```python
from build123d import *

# Parameters (mm, degrees)
SKETCH1_R                    = 14
BOSS_EXTRUDE1_DEPTH          = 10
SKETCH2_R                    = 6
CUT_EXTRUDE1_DEPTH           = 23.181073013
SKETCH3_R                    = 1.5
CUT_EXTRUDE2_DEPTH           = 23.181073013
CHAMFER1_SIZE                = 0.8
CHAMFER2_SIZE                = 0.3
CIRPATTERN1_COUNT            = 3
CHAMFER2_OF_CIRPATTERN1_SIZE = 0.3


with BuildPart() as part:
    # Sketch1 → Boss-Extrude1 (new body)
    with BuildSketch(Plane(origin=(0, 0, 0), x_dir=(1, 0, 0), z_dir=(0, 1, 0))):
        with Locations(Location((0, 0, 0), (0, 0, 270))):
            Circle(SKETCH1_R)
    extrude(amount=BOSS_EXTRUDE1_DEPTH)

    # Sketch2 → Cut-Extrude1 (cut, through all)
    with BuildSketch(Plane(origin=(0, 10, 0), x_dir=(1, 0, 0), z_dir=(0, 1, 0))):
        with Locations(Location((0, 0, 0), (0, 0, 270))):
            Circle(SKETCH2_R)
    extrude(amount=-CUT_EXTRUDE1_DEPTH, mode=Mode.SUBTRACT)

    # Sketch3 → Cut-Extrude2 (cut, through all)
    with BuildSketch(Plane(origin=(0, 10, 0), x_dir=(1, 0, 0), z_dir=(0, 1, 0))):
        with Locations(Location((0, 10.5, 0), (0, 0, 270))):
            Circle(SKETCH3_R)
    cut_extrude2 = extrude(amount=-CUT_EXTRUDE2_DEPTH, mode=Mode.SUBTRACT)

    # Chamfer1
    chamfer1_edges = [part.edges().sort_by_distance(p)[0] for p in [
        (0, 0, -14),
        (0, 10, -14),
        (0, 0, -6),
        (0, 10, -6),
    ]]
    chamfer(chamfer1_edges, length=CHAMFER1_SIZE)

    # Chamfer2
    chamfer2_edges = [part.edges().sort_by_distance(p)[0] for p in [
        (0, 0, -12),
        (0, 10, -12),
    ]]
    chamfer(chamfer2_edges, length=CHAMFER2_SIZE)

    # CirPattern1: Cut-Extrude2 ×3 about axis
    cirpattern1_axis = Axis((0, 0, 0), (0, 1, 0))
    for i in range(1, CIRPATTERN1_COUNT):
        add(cut_extrude2.rotate(cirpattern1_axis, i * 360 / CIRPATTERN1_COUNT), mode=Mode.SUBTRACT)

    # Chamfer2 of CirPattern1
    chamfer2_of_cirpattern1_edges = [part.edges().sort_by_distance(p)[0] for p in [
        (-10.392304845, 0, 6),
        (-10.392304845, 10, 6),
        (10.392304845, 0, 6),
        (10.392304845, 10, 6),
    ]]
    chamfer(chamfer2_of_cirpattern1_edges, length=CHAMFER2_OF_CIRPATTERN1_SIZE)


solid = part.part
```
Source: CAD feature listing. Evaluate the final solid. Frame: model axes, mm. Give positions to 0.01 mm unless a question says otherwise; leave off trailing zeros. Order: outer loops, then holes, each group sorted by start corner. A loop starts at its lowest first (then second) coordinate and runs counter-clockwise, first axis right, second up.
(1) Material intervals for line 1 along Z through (x, y) = (0.5, 8); line 2 along X through (y, z) = (6.25, 5.5); line 3 along Z through (x, y) = (-3.75, 6.5), sorted ascending.
(2) Section query C-C (y = 3.5). Return the cut outline in (x, z).
(3) Contact query for flat-ended pins moving along their axis: P1, Ø4, axis at y = 8.5, z = -8.5, coming from the -X side; P2, Ø2, axis at x = 6, y = 4.5, coming from the +Z side; P3, Ø3, axis at y = 2.5, z = 2, coming from the -X side; P4, Ø2.5, axis at x = 0, z = -10.5, coming from the +Y side. Output: stop coordinate, or through.
(4) Section query B-B (x = 0). Return the cut outline in (y, z), plus the area to 3 significant figures.
(5) Section query A-A (z = 0). Return the cut outline in (x, y).
(6) Section query D-D (z = 5.25). State how many separate pieces and enclosed holes the cut face has, plus the area to 3 significant figures.
(7) Pull-direction query (X, two-part tool) for faces 1 (the face through (-13.67, 4.94, -3.03)), 2 (the face through (1.802, 5.059, 5.723)), 3 (the face through (-6, 10, 6)); classes: +X half, -X half, draft (parallel to the pull), parting line (faces both ways), or undercut.
Outcome:
1. line 1: z = -13.99 to -11.91, -9.09 to -5.98, 5.98 to 13.99
1. line 2: x = -12.87 to -10.57, -7.61 to -2.4, 2.4 to 7.61, 10.57 to 12.87
1. line 3: z = -13.49 to -4.68, 4.68 to 13.49
2. outline: circle Ø28 at (0, 0); hole circle Ø3 at (-9.09, 5.25); hole circle Ø12 at (0, 0); hole circle Ø3 at (0, -10.5); hole circle Ø3 at (9.09, 5.25)
3. P1: stops at x = -12.4
3. P2: stops at z = 13.08
3. P3: stops at x = -13.99
3. P4: passes through
4. outline: (0, -13.2) - (0.8, -14) - (9.2, -14) - (10, -13.2) - (10, -12.3) - (9.7, -12) - (0.3, -12) - (0, -12.3) - close; (0, -8.7) - (0.3, -9) - (9.7, -9) - (10, -8.7) - (10, -6.8) - (9.2, -6) - (0.8, -6) - (0, -6.8) - close; (0, 6.8) - (0.8, 6) - (9.2, 6) - (10, 6.8) - (10, 13.2) - (9.2, 14) - (0.8, 14) - (0, 13.2) - close
4. area: 127 mm2
5. outline: (-14, 0.8) - (-13.2, 0) - (-6.8, 0) - (-6, 0.8) - (-6, 9.2) - (-6.8, 10) - (-13.2, 10) - (-14, 9.2) - close; (6, 0.8) - (6.8, 0) - (13.2, 0) - (14, 0.8) - (14, 9.2) - (13.2, 10) - (6.8, 10) - (6, 9.2) - close
6. separate pieces: 4
6. enclosed holes: 0
6. area: 137 mm2
7. face 1: parting line
7. face 2: undercut
7. face 3: draft
